Autodesk Fusion 360 part; units mm, degrees
sketch "Sketch1" plane through (0, 0, 0) normal (0, 0, 1) x (1, 0, 0)
  line L0 (-111, 0.4) -> (111, 0.4)
  line L1 (111, 0.4) -> (111, 44.05)
  line L2 (111, 44.05) -> (-111, 44.05)
  line L3 (-111, 44.05) -> (-111, 0.4)
extrude "Extrude1" add sketch "Sketch1" along normal blind 4
sketch "Sketch2" plane through (0, 0, 0) normal (0, 0, 1) x (1, 0, 0)
  circle A0 centre (-63.55, 22.225) radius 19.5
  circle A1 centre (-79.55, 6.225) radius 1.8
  circle A2 centre (-79.55, 38.225) radius 1.8
  circle A3 centre (-47.55, 6.225) radius 1.8
  circle A4 centre (-47.55, 38.225) radius 1.8
  circle A5 centre (0, 22.225) radius 19.5
  circle A6 centre (-16, 6.225) radius 1.8
  circle A7 centre (-16, 38.225) radius 1.8
  circle A8 centre (16, 6.225) radius 1.8
  circle A9 centre (16, 38.225) radius 1.8
  circle A10 centre (63.55, 22.225) radius 19.5
  circle A11 centre (47.55, 6.225) radius 1.8
  circle A12 centre (47.55, 38.225) radius 1.8
  circle A13 centre (79.55, 6.225) radius 1.8
  circle A14 centre (79.55, 38.225) radius 1.8
  circle A15 centre (-102.82, 15) radius 1.7
  circle A16 centre (-102.82, 29.45) radius 1.7
  circle A17 centre (102.82, 15) radius 1.7
  circle A18 centre (102.82, 29.45) radius 1.7
extrude "Extrude2" cut sketch "Sketch2" along normal blind 4
sketch "Sketch3" plane through (0, 0, 0) normal (0, 0, 1) x (1, 0, 0)
  line L0 (-90.69, 15) -> (-88.19, 15)
  line L1 (-88.19, 15) -> (-88.19, 20)
  line L2 (-88.19, 20) -> (-90.69, 20)
  line L3 (-90.69, 20) -> (-90.69, 15)
  line L4 (-90.69, 24.5) -> (-88.19, 24.5)
  line L5 (-88.19, 24.5) -> (-88.19, 29.5)
  line L6 (-88.19, 29.5) -> (-90.69, 29.5)
  line L7 (-90.69, 29.5) -> (-90.69, 24.5)
  line L8 (-33.03, 15) -> (-30.53, 15)
  line L9 (-30.53, 15) -> (-30.53, 20)
  line L10 (-30.53, 20) -> (-33.03, 20)
  line L11 (-33.03, 20) -> (-33.03, 15)
  line L12 (-33.03, 24.5) -> (-30.53, 24.5)
  line L13 (-30.53, 24.5) -> (-30.53, 29.5)
  line L14 (-30.53, 29.5) -> (-33.03, 29.5)
  line L15 (-33.03, 29.5) -> (-33.03, 24.5)
  line L16 (30.53, 15) -> (33.03, 15)
  line L17 (33.03, 15) -> (33.03, 20)
  line L18 (33.03, 20) -> (30.53, 20)
  line L19 (30.53, 20) -> (30.53, 15)
  line L20 (30.53, 24.5) -> (33.03, 24.5)
  line L21 (33.03, 24.5) -> (33.03, 29.5)
  line L22 (33.03, 29.5) -> (30.53, 29.5)
  line L23 (30.53, 29.5) -> (30.53, 24.5)
  line L24 (88.19, 15) -> (90.69, 15)
  line L25 (90.69, 15) -> (90.69, 20)
  line L26 (90.69, 20) -> (88.19, 20)
  line L27 (88.19, 20) -> (88.19, 15)
  line L28 (88.19, 24.5) -> (90.69, 24.5)
  line L29 (90.69, 24.5) -> (90.69, 29.5)
  line L30 (90.69, 29.5) -> (88.19, 29.5)
  line L31 (88.19, 29.5) -> (88.19, 24.5)
extrude "Extrude3" cut sketch "Sketch3" along normal blind 4
ref_plane "WorkPlane1" through (0, 0, 4) normal (0, 0, 1) x (1, 0, 0)
sketch "Sketch4" plane through (0, 0, 4) normal (0, 0, 1) x (1, 0, 0)
  circle A0 centre (-102.82, 15) radius 3.25
  circle A1 centre (-102.82, 29.45) radius 3.25
  circle A2 centre (102.82, 15) radius 3.25
  circle A3 centre (102.82, 29.45) radius 3.25
extrude "Extrude4" cut sketch "Sketch4" against normal blind 2
sketch "Sketch5" plane through (0, 0, 0) normal (0, 0, 1) x (1, 0, 0)
  line L0 (-97.6, 2) -> (97.6, 2)
  line L1 (97.6, 2) -> (97.6, 4.4)
  line L2 (97.6, 4.4) -> (-97.6, 4.4)
  line L3 (-97.6, 4.4) -> (-97.6, 2)
  line L4 (-97.6, 40.05) -> (97.6, 40.05)
  line L5 (97.6, 40.05) -> (97.6, 42.45)
  line L6 (97.6, 42.45) -> (-97.6, 42.45)
  line L7 (-97.6, 42.45) -> (-97.6, 40.05)
extrude "Extrude5" cut sketch "Sketch5" along normal blind 2
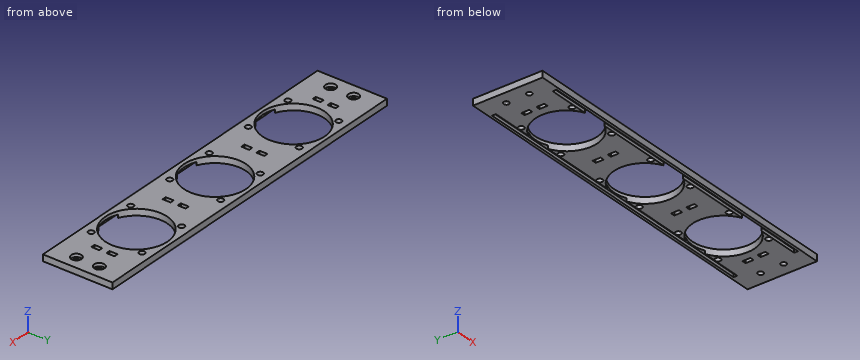
Work out the finished part from the listing and answer in its coordinate system (mm). Give positions to 0.01 mm unless a question says otherwise; leave off trailing zeros. Loops run counter-clockwise (first coordinate to the right, second up) from the corner with the lowest first, then second, coordinate; pieces in that order, holes last. Notation, with made-up numbers: M -27,72 L 8,72 A22 ccw 8,88 Z; hole C 41,-24.5 d11. An arc over 180 degrees is marked long. One line per item, written item: value. Start each with the question number.
1. Find section C-C (z = 3). State how many separate pieces and enclosed holes the cut face has, and give its area (3 significant figures).
2. Find section A-A (x = 63.55). Give the vertices of the cut face in (y, z) (3 decimals), and give its area (3 significant figures).
3. Find section B-B (x = 95). Give the vertices of the cut face in (y, z).
4. Find the intervals of material crossed by probe 1 along Y at (x, z) = (-102.82, 2.85); probe 2 along Y at (x, z) = (83.5, 1.8); probe 3 along Y at (x, z) = (-63.55, 3.05) (3 decimals), in increasing order.
5. Find section D-D (x = 5.5). Give the vertices of the cut face in (y, z).
Reported:
1. separate pieces: 1
1. enclosed holes: 27
1. area: 5,750 mm²
2. outline: M 0.4,0 L 2,0 L 2,2 L 2.725,2 L 2.725,4 L 0.4,4 Z; M 41.725,2 L 42.45,2 L 42.45,0 L 44.05,0 L 44.05,4 L 41.725,4 Z
2. area: 15.7 mm²
3. outline: M 0.4,0 L 2,0 L 2,2 L 4.4,2 L 4.4,0 L 40.05,0 L 40.05,2 L 42.45,2 L 42.45,0 L 44.05,0 L 44.05,4 L 0.4,4 Z
4. probe 1: y = 0.4 to 11.75, 18.25 to 26.2, 32.7 to 44.05
4. probe 2: y = 0.4 to 2, 4.4 to 40.05, 42.45 to 44.05
4. probe 3: y = 0.4 to 2.725, 41.725 to 44.05
5. outline: M 0.4,0 L 2,0 L 2,2 L 3.52,2 L 3.52,4 L 0.4,4 Z; M 40.93,2 L 42.45,2 L 42.45,0 L 44.05,0 L 44.05,4 L 40.93,4 Z
